Read the model definition and answer for the solid it produces. Units are mm, in the model's axes. A direction names the side the tool comes from. Coordinates: 2 decimals unless noted, no trailing zeros. Loops run counter-clockwise (first coordinate to the right, second up) from the corner with the lowest first, then second, coordinate; pieces in that order, holes last.
Autodesk Inventor part; units mm, degrees
ref_plane "YZ Plane" through (0, 0, 0) normal (1, 0, 0) x (0, 1, 0)
ref_plane "XZ Plane" through (0, 0, 0) normal (0, 1, 0) x (-1, 0, 0)
ref_plane "XY Plane" through (0, 0, 0) normal (0, 0, 1) x (1, 0, 0)
sketch "Sketch1" plane through (0, 0, 0) normal (0, 1, 0) x (-1, 0, 0)
  circle A0 centre (0, 0) radius 2.5
  circle A1 centre (0, 0) radius 4
  circle A2 centre (-30, 0) radius 2.5
  circle A3 centre (-30, 0) radius 4
  line L0 (0, 2.5) -> (-30, 2.5)
  line L1 (-30, 2.5) -> (-30, -2.5)
  line L2 (-30, -2.5) -> (0, -2.5)
  line L3 (0, -2.5) -> (0, 2.5)
  point P0 (-3.4641, 2)
  point P1 (-26.5359, 2)
  point P2 (-26.5359, -2)
  point P3 (-3.4641, -2)
  point P4 (-27.2006, 2.8571)
  point P5 (-2.7994, 2.8571)
  point P6 (-2.7994, -2.8571)
  point P7 (-27.2006, -2.8571)
  point P8 (-26.8775, -2.5)
  point P9 (-3.1225, -2.5)
  point P10 (-3.1225, 2.5)
  point P11 (-26.8775, 2.5)
  dimension "d0" = 5
  dimension "d2" = 5
  dimension "d1" = 8
  dimension "d3" = 8
  dimension "d4" = 30
extrude "Extrusion1" add sketch "Sketch1" along normal blind 3 contours A0 L0 A1 L2 | A0 L2 A1 L0 | A1 L2 A3 L0 | L0 A2 L2 A3 | A3 L2 A2 L0
extrude "Extrusion2" add sketch "Sketch1" against normal blind 3 contours L0 A2 L2 A3 | A3 L2 A2 L0
properties part number "Arm Link_3DPrint"
Q1. A cutting plane is placed at B-B (z = -2). Give the vertices of the cut face in (x, y), then the cut area to 3 significant figures.
Findings below:
outline: (-3.46, 0) - (-1.5, 0) - (-1.5, 3) - (-3.46, 3) - close; (1.5, 0) - (26.54, 0) - (26.54, -3) - (28.5, -3) - (28.5, 3) - (1.5, 3) - close; (31.5, -3) - (33.46, -3) - (33.46, 3) - (31.5, 3) - close
area: 105 mm2
Q2. Straight lines are drawn through the part: probe 1 along X at (y, z) = (1.7, 0); probe 2 along Z at (x, y) = (0, 1.4); probe 3 along X at (y, z) = (0.6, 1.75). For each, find the intervals that lie inside material, in ascending order.
Findings below:
probe 1: x = -4 to -2.5, 2.5 to 27.5, 32.5 to 34
probe 2: z = -4 to -2.5, 2.5 to 4
probe 3: x = -3.6 to -1.79, 1.79 to 28.21, 31.79 to 33.6
Q3. Determine the mould class of faces 1 (the face through (15, 1, 2.5)), 2 (the face through (0.54, 1.48, 2.44)), 3 (the face through (34, 0, 0)) for opening direction Z: +Z half, -Z half, draft (parallel to the pull), parting line (faces both ways), or undercut.
Findings below:
face 1: +Z half
face 2: undercut
face 3: parting line
Q4. A cutting plane is placed at D-D (x = 30). Give the vertices of the cut face in (y, z).
Findings below:
outline: (-3, -4) - (3, -4) - (3, -2.5) - (-3, -2.5) - close; (-3, 2.5) - (3, 2.5) - (3, 4) - (-3, 4) - close
Q5. A cutting plane is placed at C-C (y = 2.4). Give the vertices of the cut face in (x, z), then the cut area to 3 significant figures.
Findings below:
outline: (3.12, -2.5) - (26.88, -2.5) arc R4 ccw (long way) to (26.88, 2.5) - (3.12, 2.5) arc R4 ccw (long way) to start; hole circle Ø5 at (0, 0); hole circle Ø5 at (30, 0)
area: 174 mm2
Q6. A cutting plane is placed at A-A (x = 0). Give the vertices of the cut face in (y, z), then the cut area to 3 significant figures.
Findings below:
outline: (0, -4) - (3, -4) - (3, -2.5) - (0, -2.5) - close; (0, 2.5) - (3, 2.5) - (3, 4) - (0, 4) - close
area: 9.00 mm2
Q7. Flat-ended cylindrical pins translate along their axes: pin 1 Ø3.5 at (x, y) = (17, 1) entering from -Z; pin 2 Ø3.5 at (x, y) = (11.5, 1) entering from +Z; pin 3 Ø2 at (y, z) = (1, 1.5) entering from -X. Find the tip coordinate at first contact, or state that the pin passes through.
Findings below:
pin 1: stops at z = -2.5
pin 2: stops at z = 2.5
pin 3: stops at x = -3.97
Q8. Which of the six approach directions +Z, -Z, +X, -X, +Y, -Y give full straight-line access (tool end or side, diameter ignored) to faces 4 (the face through (32.5, 0, -0.1)), 5 (the face through (15, 1, -2.5))?
Findings below:
face 4: +Y, -Y
face 5: -Z, +Y, -Y
